The listing builds one solid part. Answer for the finished solid, in the listing's coordinates (mm). Coordinates: 2 decimals unless noted, no trailing zeros. Order: outer loops, then holes, each group sorted by start corner. A loop starts at its lowest first (then second) coordinate and runs counter-clockwise, first axis right, second up.
```python
from build123d import *

# Parameters (mm, degrees)
SKETCH1_R           = 76.2
BOSS_EXTRUDE1_DEPTH = 6.35
SKETCH2_R           = 1.905
CUT_EXTRUDE1_DEPTH  = 108.95
SKETCH3_R           = 3.429
CUT_EXTRUDE2_DEPTH  = 108.95
SKETCH4_R           = 6.35
CUT_EXTRUDE3_DEPTH  = 108.95
SKETCH5_R           = 6.35
CUT_EXTRUDE4_DEPTH  = 108.95
SKETCH7_R           = 2.54
CUT_EXTRUDE6_DEPTH  = 108.95
SKETCH8_R           = 3.429
CUT_EXTRUDE7_DEPTH  = 108.95
SKETCH9_R           = 3.429
CUT_EXTRUDE8_DEPTH  = 108.95
SKETCH10_R          = 2.54
BOSS_EXTRUDE2_DEPTH = 6.35
SKETCH11_R          = 2.286
CUT_EXTRUDE9_DEPTH  = 108.95


with BuildPart() as part:
    # Sketch1 → Boss-Extrude1 (new body)
    with BuildSketch(Plane(origin=(0, 0, 0), x_dir=(1, 0, 0), z_dir=(0, 1, 0))):
        with Locations(Location((0, 0, 0), (0, 0, 270))):
            Circle(SKETCH1_R)
    extrude(amount=BOSS_EXTRUDE1_DEPTH)

    # Sketch2 → Cut-Extrude1 (cut, through all)
    with BuildSketch(Plane(origin=(0, 6.35, 0), x_dir=(1, 0, 0), z_dir=(0, 1, 0))):
        with Locations(Location((0, 0, 0), (0, 0, 270))):
            Circle(SKETCH2_R)
    extrude(amount=-CUT_EXTRUDE1_DEPTH, mode=Mode.SUBTRACT)

    # Sketch3 → Cut-Extrude2 (cut, through all)
    with BuildSketch(Plane(origin=(0, 6.35, 0), x_dir=(1, 0, 0), z_dir=(0, 1, 0))):
        with Locations(Location((0, 14.732, 0), (0, 0, 270))):
            Circle(SKETCH3_R)
        with Locations(Location((-13.97, -10.631143259, 0), (0, 0, 270))):
            Circle(SKETCH3_R)
        with Locations(Location((13.97, -10.631143259, 0), (0, 0, 270))):
            Circle(SKETCH3_R)
    extrude(amount=-CUT_EXTRUDE2_DEPTH, mode=Mode.SUBTRACT)

    # Sketch4 → Cut-Extrude3 (cut, through all)
    with BuildSketch(Plane(origin=(0, 6.35, 0), x_dir=(1, 0, 0), z_dir=(0, 1, 0))):
        with Locations(Location((-25.4, -50.8, 0), (0, 0, 270))):
            Circle(SKETCH4_R)
        with Locations(Location((25.4, -50.8, 0), (0, 0, 270))):
            Circle(SKETCH4_R)
    extrude(amount=-CUT_EXTRUDE3_DEPTH, mode=Mode.SUBTRACT)

    # Sketch5 → Cut-Extrude4 (cut, through all)
    with BuildSketch(Plane(origin=(0, 6.35, 0), x_dir=(1, 0, 0), z_dir=(0, 1, 0))):
        with Locations(Location((-25.4, 50.8, 0), (0, 0, 270))):
            Circle(SKETCH5_R)
        with Locations(Location((25.4, 50.8, 0), (0, 0, 270))):
            Circle(SKETCH5_R)
    extrude(amount=-CUT_EXTRUDE4_DEPTH, mode=Mode.SUBTRACT)

    # Sketch7 → Cut-Extrude6 (cut, through all)
    with BuildSketch(Plane(origin=(0, 6.35, 0), x_dir=(1, 0, 0), z_dir=(0, 1, 0))):
        with Locations(Location((0, 46.99, 0), (0, 0, 270))):
            Circle(SKETCH7_R)
        with Locations(Location((0, -46.99, 0), (0, 0, 270))):
            Circle(SKETCH7_R)
    extrude(amount=-CUT_EXTRUDE6_DEPTH, mode=Mode.SUBTRACT)

    # Sketch8 → Cut-Extrude7 (cut, through all)
    with BuildSketch(Plane(origin=(0, 6.35, 0), x_dir=(1, 0, 0), z_dir=(0, 1, 0))):
        with Locations(Location((57.15, 0, 0), (0, 0, 270))):
            Circle(SKETCH8_R)
    extrude(amount=-CUT_EXTRUDE7_DEPTH, mode=Mode.SUBTRACT)

    # Sketch9 → Cut-Extrude8 (cut, through all)
    with BuildSketch(Plane(origin=(0, 6.35, 0), x_dir=(1, 0, 0), z_dir=(0, 1, 0))):
        with Locations(Location((-48.26, -31.75, 0), (0, 0, 270))):
            Circle(SKETCH9_R)
        with Locations(Location((-48.26, 31.75, 0), (0, 0, 270))):
            Circle(SKETCH9_R)
    extrude(amount=-CUT_EXTRUDE8_DEPTH, mode=Mode.SUBTRACT)

    # Sketch10 → Boss-Extrude2 (add)
    with BuildSketch(Plane(origin=(0, 6.35, 0), x_dir=(1, 0, 0), z_dir=(0, 1, 0))):
        with Locations((0, 46.99)):
            Circle(SKETCH10_R)
        with Locations((0, -46.99)):
            Circle(SKETCH10_R)
    extrude(amount=-BOSS_EXTRUDE2_DEPTH)

    # Sketch11 → Cut-Extrude9 (cut, through all)
    with BuildSketch(Plane(origin=(0, 6.35, 0), x_dir=(1, 0, 0), z_dir=(0, 1, 0))):
        with Locations(Location((0, -31.75, 0), (0, 0, 270))):
            Circle(SKETCH11_R)
        with Locations(Location((0, 31.75, 0), (0, 0, 270))):
            Circle(SKETCH11_R)
    extrude(amount=-CUT_EXTRUDE9_DEPTH, mode=Mode.SUBTRACT)


solid = part.part
```
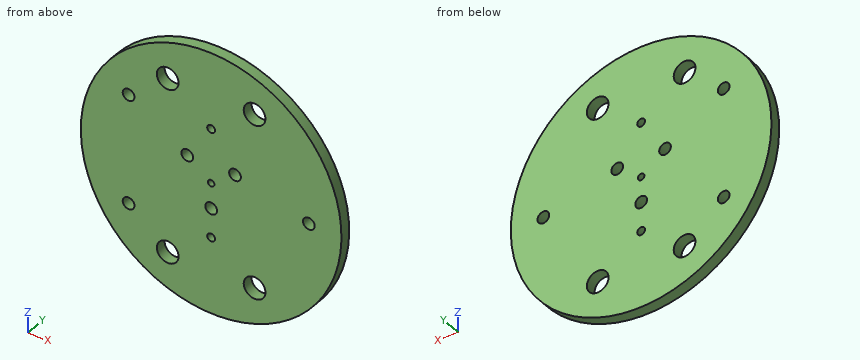
1) This flat-tipped pin is pushed along its axis until it touches: P1, Ø1.5, axis at y = 3.5, z = -24, coming from the -X side. Where does it stop, or does it pass through?
2) A cutting plane is placed at B-B, the plane y = 1. Count the separate pieces of the cut face and the enclosed holes in it, plus the area to 3 significant figures.
3) A cutting plane is placed at D-D, the plane x = -13.97. Write down the section's boundary in (y, z).
4) A cutting plane is placed at A-A, the plane z = 31.75. Write down the section's boundary in (x, y), plus the area to 3 significant figures.
5) A cutting plane is placed at C-C, the plane x = -48.26. Write down the section's boundary in (y, z).
6) Straight lines are drawn through the part: probe 1 along Z at (x, y) = (-0.5, 4.75); probe 2 along X at (y, z) = (1.5, -31.75); probe 3 along X at (y, z) = (5.5, 9.5). For each, find the intervals that lie inside material, in ascending order.
Working result:
1. P1: stops at x = -72.57
2. separate pieces: 1
2. enclosed holes: 13
2. area: 17,500 mm2
3. outline: (0, -74.91) - (6.35, -74.91) - (6.35, 7.2) - (0, 7.2) - close; (0, 14.06) - (6.35, 14.06) - (6.35, 74.91) - (0, 74.91) - close
4. outline: (-69.27, 0) - (-51.69, 0) - (-51.69, 6.35) - (-69.27, 6.35) - close; (-44.83, 0) - (-2.29, 0) - (-2.29, 6.35) - (-44.83, 6.35) - close; (2.29, 0) - (69.27, 0) - (69.27, 6.35) - (2.29, 6.35) - close
4. area: 807 mm2
5. outline: (0, -58.97) - (6.35, -58.97) - (6.35, -35.18) - (0, -35.18) - close; (0, -28.32) - (6.35, -28.32) - (6.35, 28.32) - (0, 28.32) - close; (0, 35.18) - (6.35, 35.18) - (6.35, 58.97) - (0, 58.97) - close
6. probe 1: z = -76.2 to -33.98, -29.52 to -18.12, -11.34 to -1.84, 1.84 to 29.52, 33.98 to 76.2
6. probe 2: x = -69.27 to -51.69, -44.83 to -2.29, 2.29 to 69.27
6. probe 3: x = -75.61 to -17.21, -10.73 to 10.73, 17.21 to 75.61
